Design review of the part built by this model. Coordinates are the model's own, in mm. Face numbers are marked on the shaded views. Give positions to 0.01 mm unless a question says otherwise; leave off trailing zeros. Loops run counter-clockwise (first coordinate to the right, second up) from the corner with the lowest first, then second, coordinate; pieces in that order, holes last. Notation, with made-up numbers: (54, 36) - (68, 36) arc R24 cw to (68, 61) - close; hole circle Ø11 at (47, 4). An arc over 180 degrees is marked (long way). One line per item, written item: value. Start each with the question number.
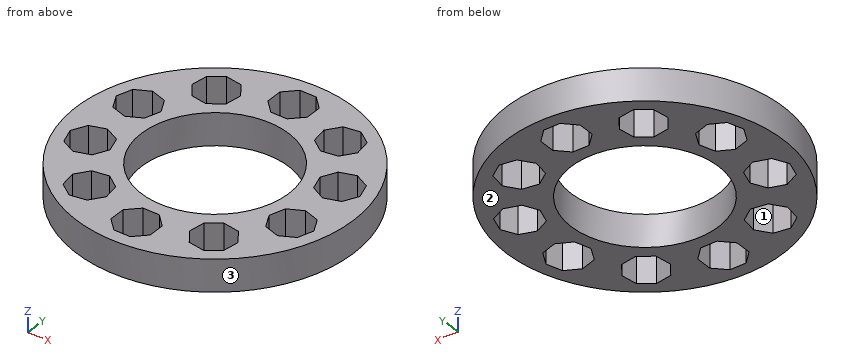
```python
from build123d import *

# Parameters (mm, degrees)
CROQUIS1_R              = 19
CROQUIS1_R_2            = 10.1
SALIENTE_EXTRUIR1_DEPTH = 4.4
CORTAR_EXTRUIR1_DEPTH   = 4.4
MATRIZC1_COUNT          = 10


with BuildPart() as part:
    # Croquis1 → Saliente-Extruir1 (new body)
    with BuildSketch(Plane(origin=(0, 0, 0), x_dir=(0, 1, 0), z_dir=(0, 0, 1))):
        with Locations(Location((0, 0, 0), (0, 0, 270))):
            Circle(CROQUIS1_R)
        with Locations(Location((0, 0, 0), (0, 0, 270))):
            Circle(CROQUIS1_R_2, mode=Mode.SUBTRACT)
    extrude(amount=SALIENTE_EXTRUIR1_DEPTH)

    # Croquis2 → Cortar-Extruir1 (cut)
    with BuildSketch(Plane.XY.offset(4.4)):
        Polygon((2.7, 13.431623382), (2.7, 15.668376618), (1.118376618, 17.25), (-1.118376618, 17.25), (-2.7, 15.668376618), (-2.7, 13.431623382), (-1.118376618, 11.85), (1.118376618, 11.85), align=None)
    cortar_extruir1 = extrude(amount=-CORTAR_EXTRUIR1_DEPTH, mode=Mode.SUBTRACT)

    # MatrizC1: Cortar-Extruir1 ×10 about axis
    matrizc1_axis = Axis((0, 0, 0), (0, 0, 1))
    for i in range(1, MATRIZC1_COUNT):
        add(cortar_extruir1.rotate(matrizc1_axis, i * 360 / MATRIZC1_COUNT), mode=Mode.SUBTRACT)


solid = part.part
```
(1) For pin 1 Ø3 at (x, y) = (6.5, 4) entering from +Z; pin 2 Ø1.1 at (y, z) = (-14.5, 2.5) entering from -X; pin 3 Ø1.8 at (x, z) = (-0.5, 1) entering from -Y; pin 4 Ø2 at (y, z) = (-6, 2.5) entering from -X, all flat-tipped, find the tip position at first contact; note any pin that passes through.
(2) To check wall thickness, follow L1, parallel to Y at x = 0, z = 1.85; L2, parallel to X at y = 4, z = 3.2; L3, parallel to Y at x = 12, z = 0.35. State the ranges of each line that lie inside material, in increasing order. Write a range as from..to.
(3) Draft analysis for pull direction X (two halves, no side actions). For the marked faces 1, 2 and 3, state which applies: pulls with the +X half, pulls with the -X half, needs draft (parallel to the pull), parting line crosses it, or undercut.
(4) Take a section at C-C on x = 5. State the section outline as (y, z) points.
(5) Take a section at B-B on x = 0. State the section outline as (y, z) points, and give its area (3 significant figures).
(6) Take a section at A-A on y = 0. State the section outline as (x, z) points.
(7) Take a section at D-D on z = 3.8. State how many separate pieces and enclosed holes the cut face has, and give its area (3 significant figures).
Here are the results:
1. pin 1: through
1. pin 2: x = -12.9
1. pin 3: y = -19
1. pin 4: x = -18.33
2. L1: -19..-17.25, -11.85..-10.1, 10.1..11.85, 17.25..19
2. L2: -18.57..-16.62, -11.16..-9.27, 9.27..11.16, 16.62..18.57
2. L3: -14.73..-6.74, -2.4..2.4, 6.74..14.73
3. face 1: undercut
3. face 2: needs draft
3. face 3: parting line crosses it
4. outline: (-18.33, 0) - (-8.78, 0) - (-8.78, 4.4) - (-18.33, 4.4) - close; (8.78, 0) - (18.33, 0) - (18.33, 4.4) - (8.78, 4.4) - close
5. outline: (-19, 0) - (-17.25, 0) - (-17.25, 4.4) - (-19, 4.4) - close; (-11.85, 0) - (-10.1, 0) - (-10.1, 4.4) - (-11.85, 4.4) - close; (10.1, 0) - (11.85, 0) - (11.85, 4.4) - (10.1, 4.4) - close; (17.25, 0) - (19, 0) - (19, 4.4) - (17.25, 4.4) - close
5. area: 30.8 mm²
6. outline: (-19, 0) - (-10.1, 0) - (-10.1, 4.4) - (-19, 4.4) - close; (10.1, 0) - (19, 0) - (19, 4.4) - (10.1, 4.4) - close
7. separate pieces: 1
7. enclosed holes: 11
7. area: 572 mm²
